Geometry: final body of the model. Coordinates: model frame, mm. Face numbers are marked on the shaded views. A direction names the side the tool comes from. Coordinates: 2 decimals unless noted, no trailing zeros. Order: outer loops, then holes, each group sorted by start corner. A loop starts at its lowest first (then second) coordinate and runs counter-clockwise, first axis right, second up. Notation, with made-up numbers: (-18, 79.25) - (11, 79.25) arc R34 ccw to (11, 116.25) - close; hole circle Ø8 at (-23.75, 87). An arc over 180 degrees is marked (long way). Use a Markdown table: item, result. Add a question column.
```python
from build123d import *

# Parameters (mm, degrees)
SKETCH1_W                                  = 128
SKETCH1_H                                  = 105
BOSS_EXTRUDE1_DEPTH                        = 3
SKETCH2_W                                  = 13.5
SKETCH2_H                                  = 105
BOSS_EXTRUDE2_DEPTH                        = 2.9
BOSS_EXTRUDE9_DEPTH                        = 7
FILLET2_R                                  = 1
CUT_EXTRUDE1_DEPTH                         = 7
SKETCH3_W                                  = 3
SKETCH3_H                                  = 95
BOSS_EXTRUDE10_DEPTH                       = 20
SKETCH11_R                                 = 1
CUT_EXTRUDE2_DEPTH                         = 20
SKETCH13_R                                 = 1
CUT_EXTRUDE3_DEPTH                         = 20
MIRROR1_AT_THE_SECOND_PLANE_COPY_1_SKETC_R = 1
MIRROR1_AT_THE_SECOND_PLANE_COPY_1_DEPTH   = 20
CUT_EXTRUDE8_DEPTH                         = 5
FILLET3_R                                  = 10


with BuildPart() as part:
    # Sketch1 → Boss-Extrude1 (new body)
    with BuildSketch(Plane(origin=(0, 0, 0), x_dir=(1, 0, 0), z_dir=(0, 1, 0))):
        Rectangle(SKETCH1_W, SKETCH1_H)
    extrude(amount=BOSS_EXTRUDE1_DEPTH)

    # Sketch2 → Boss-Extrude2 (add)
    with BuildSketch(Plane(origin=(0, 0, 0), x_dir=(1, 0, 0), z_dir=(0, 1, 0))):
        with Locations((-70.75, 0)):
            Rectangle(SKETCH2_W, SKETCH2_H)
        with Locations((70.75, 0)):
            Rectangle(SKETCH2_W, SKETCH2_H)
    extrude(amount=BOSS_EXTRUDE2_DEPTH)

    # Sketch5 → Boss-Extrude9 (add)
    with BuildSketch(Plane(origin=(0, 3, 0), x_dir=(1, 0, 0), z_dir=(0, 1, 0))):
        Polygon((-6, -18.5), (-6, -17.5), (-13, -17.5), (-13, 17.5), (13, 17.5), (13, -17.5), (6, -17.5), (6, -18.5), (14, -18.5), (14, 18.5), (-14, 18.5), (-14, -18.5), align=None)
    extrude(amount=BOSS_EXTRUDE9_DEPTH)

    # Fillet2
    fillet2_edges = [part.edges().sort_by_distance(p)[0] for p in [
        (13, 6.5, 17.5),
        (14, 6.5, 18.5),
        (14, 6.5, -18.5),
        (-14, 6.5, -18.5),
        (-14, 6.5, 18.5),
        (-13, 6.5, 17.5),
        (-13, 6.5, -17.5),
        (13, 6.5, -17.5),
    ]]
    fillet(fillet2_edges, radius=FILLET2_R)

    # Sketch10 → Cut-Extrude1 (cut)
    with BuildSketch(Plane(origin=(0, 3, 0), x_dir=(1, 0, 0), z_dir=(0, 1, 0))):
        with BuildLine():
            Line((-14, -17.381354556), (-45.915455387, -42.5))
            Line((-45.915455387, -42.5), (-6, -42.5))
            Line((-6, -42.5), (-6, -18.5))
            Line((-6, -18.5), (-13, -18.5))
            ThreePointArc((-13, -18.5), (-13.707106781, -18.207106781), (-14, -17.5))
            Line((-14, -17.5), (-14, -17.381354556))
        make_face()
        Polygon((-54, -6), (-54, -36.137163962), (-15.708074024, -6), align=None)
        with BuildLine():
            Line((6, -18.5), (6, -42.5))
            Line((6, -42.5), (45.915455387, -42.5))
            Line((45.915455387, -42.5), (14, -17.381354556))
            Line((14, -17.381354556), (14, -17.5))
            ThreePointArc((14, -17.5), (13.707106781, -18.207106781), (13, -18.5))
            Line((13, -18.5), (6, -18.5))
        make_face()
        Polygon((-54, 36.137163962), (-54, 6), (-15.708074024, 6), align=None)
        Polygon((15.708074024, -6), (54, -36.137163962), (54, -6), align=None)
        with BuildLine():
            Line((-6, 42.5), (-45.915455387, 42.5))
            Line((-45.915455387, 42.5), (-14, 17.381354556))
            Line((-14, 17.381354556), (-14, 17.5))
            ThreePointArc((-14, 17.5), (-13.707106781, 18.207106781), (-13, 18.5))
            Line((-13, 18.5), (-6, 18.5))
            Line((-6, 18.5), (-6, 42.5))
        make_face()
        Polygon((15.708074024, 6), (54, 6), (54, 36.137163962), align=None)
        with BuildLine():
            Line((45.915455387, 42.5), (6, 42.5))
            Line((6, 42.5), (6, 18.5))
            Line((6, 18.5), (13, 18.5))
            ThreePointArc((13, 18.5), (13.707106781, 18.207106781), (14, 17.5))
            Line((14, 17.5), (14, 17.381354556))
            Line((14, 17.381354556), (45.915455387, 42.5))
        make_face()
    extrude(amount=-CUT_EXTRUDE1_DEPTH, mode=Mode.SUBTRACT)

    # Sketch3 → Boss-Extrude10 (add)
    with BuildSketch(Plane(origin=(0, 0, 0), x_dir=(1, 0, 0), z_dir=(0, 1, 0))):
        with Locations((-79, 0)):
            Rectangle(SKETCH3_W, SKETCH3_H)
        with Locations((79, 0)):
            Rectangle(SKETCH3_W, SKETCH3_H)
    extrude(amount=BOSS_EXTRUDE10_DEPTH)

    # Sketch11 → Cut-Extrude2 (cut)
    with BuildSketch(Plane(origin=(0, 3, 0), x_dir=(1, 0, 0), z_dir=(0, 1, 0))):
        with Locations(Location((-63.3, -41, 0), (0, 0, 270))):
            Circle(SKETCH11_R)
        with Locations(Location((-63.3, -34.5, 0), (0, 0, 270))):
            Circle(SKETCH11_R)
        with Locations(Location((-63.3, 34.5, 0), (0, 0, 270))):
            Circle(SKETCH11_R)
        with Locations(Location((-63.3, 41, 0), (0, 0, 270))):
            Circle(SKETCH11_R)
        with Locations(Location((63.3, 41, 0), (0, 0, 270))):
            Circle(SKETCH11_R)
        with Locations(Location((63.3, 34.5, 0), (0, 0, 270))):
            Circle(SKETCH11_R)
        with Locations(Location((63.3, -34.5, 0), (0, 0, 270))):
            Circle(SKETCH11_R)
        with Locations(Location((63.3, -41, 0), (0, 0, 270))):
            Circle(SKETCH11_R)
    extrude(amount=-CUT_EXTRUDE2_DEPTH, mode=Mode.SUBTRACT)

    # Sketch13 → Cut-Extrude3 (cut)
    with BuildSketch(Plane(origin=(-77.5, 0, 0), x_dir=(0, 0, -1), z_dir=(1, 0, 0))):
        with Locations((-41, 14.842473729)):
            Circle(SKETCH13_R)
        with Locations((-34.5, 14.842473729)):
            Circle(SKETCH13_R)
    cut_extrude3 = extrude(amount=-CUT_EXTRUDE3_DEPTH, mode=Mode.SUBTRACT)

    # Mirror1: Cut-Extrude3 across plane
    add(cut_extrude3.mirror(Plane.XY), mode=Mode.SUBTRACT)

    # Mirror1 at the second plane: Cut-Extrude3 across plane
    add(cut_extrude3.mirror(Plane(origin=(0, 0, 0), x_dir=(0, 0, 1), z_dir=(1, 0, 0))), mode=Mode.SUBTRACT)

    # Mirror1 at the second plane copy 1 sketc → Mirror1 at the second plane copy 1 (cut)
    with BuildSketch(Plane.ZY.offset(-77.5)):
        with Locations((-41, 14.842473729)):
            Circle(MIRROR1_AT_THE_SECOND_PLANE_COPY_1_SKETC_R)
        with Locations((-34.5, 14.842473729)):
            Circle(MIRROR1_AT_THE_SECOND_PLANE_COPY_1_SKETC_R)
    extrude(amount=-MIRROR1_AT_THE_SECOND_PLANE_COPY_1_DEPTH, mode=Mode.SUBTRACT)

    # Sketch22 → Cut-Extrude8 (cut)
    with BuildSketch(Plane(origin=(0, 10, 0), x_dir=(1, 0, 0), z_dir=(0, 1, 0))):
        with BuildLine():
            Line((14, -17.5), (14, 17.5))
            ThreePointArc((14, 17.5), (13.707106781, 18.207106781), (13, 18.5))
            Line((13, 18.5), (-13, 18.5))
            ThreePointArc((-13, 18.5), (-13.707106781, 18.207106781), (-14, 17.5))
            Line((-14, 17.5), (-14, -17.5))
            ThreePointArc((-14, -17.5), (-13.707106781, -18.207106781), (-13, -18.5))
            Line((-13, -18.5), (-6, -18.5))
            Line((-6, -18.5), (-6, -17.5))
            Line((-6, -17.5), (-12, -17.5))
            ThreePointArc((-12, -17.5), (-12.707106781, -17.207106781), (-13, -16.5))
            Line((-13, -16.5), (-13, 16.5))
            ThreePointArc((-13, 16.5), (-12.707106781, 17.207106781), (-12, 17.5))
            Line((-12, 17.5), (12, 17.5))
            ThreePointArc((12, 17.5), (12.707106781, 17.207106781), (13, 16.5))
            Line((13, 16.5), (13, -16.5))
            ThreePointArc((13, -16.5), (12.707106781, -17.207106781), (12, -17.5))
            Line((12, -17.5), (6, -17.5))
            Line((6, -17.5), (6, -18.5))
            Line((6, -18.5), (13, -18.5))
            ThreePointArc((13, -18.5), (13.707106781, -18.207106781), (14, -17.5))
        make_face()
    extrude(amount=-CUT_EXTRUDE8_DEPTH, mode=Mode.SUBTRACT)

    # Fillet3
    # the kernel refuses this fillet: 10 mm, written as the material it takes off along each edge
    with BuildSketch(Plane(origin=(6, 5, 2.5), x_dir=(0, -1, 0), z_dir=(0, 0, 1)), Plane(origin=(-6, 5, 33.5), x_dir=(0, -1, 0), z_dir=(0, 0, -1))) as fillet3_piece_1:
        with BuildLine():
            CenterArc((10, 6), FILLET3_R, 180, 36.869897646)
            Line((0, 6), (-0.2, 6))
            Line((-0.2, 6), (-0.2, 0))
            Line((-0.2, 0), (0, -0.2))
            ThreePointArc((0, -0.2), (1, -0.2), (1.84, -0.12))
            Line((1.84, -0.12), (2, 0))
        make_face()
    extrude(amount=31, mode=Mode.SUBTRACT)


solid = part.part
```
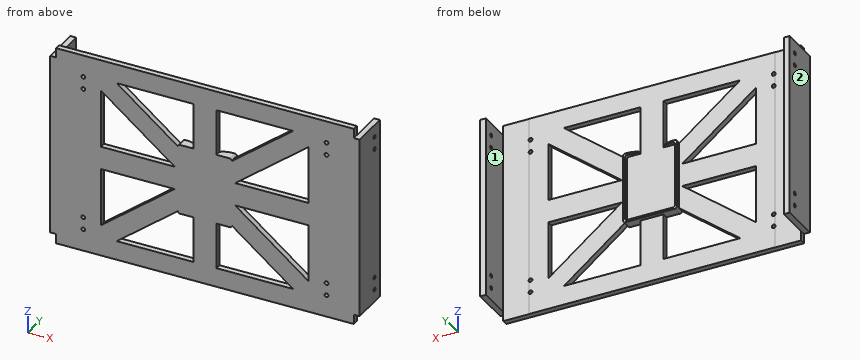
1) Pin query (flat end, axial travel): pin 1 (2.5 mm diameter, centred on x = -79.5, y = 9.5, fed in from +Z); pin 2 (1 mm diameter, centred on x = 55, z = 35.5, fed in from -Y); pin 3 (3 mm diameter, centred on y = 1, z = -50, fed in from -X); pin 4 (1.5 mm diameter, centred on x = 78.5, y = 8, fed in from -Z). Return the tip coordinate at first contact, or that it passes through.
2) Ray query, line 1 along Z through (x, y) = (-63.3, 1.65); line 2 along X through (y, z) = (11.25, -28.5); line 3 along Y through (x, z) = (78.45, 34.5). Return the intervals inside material, ascending.
3) Section A-A (y = 18). Return loops of the section in (x, z).
4) Section C-C (z = -3). Return loops of the section in (x, y), then the cut area to 3 significant figures.
5) Section D-D (z = -22). Return loops of the section in (x, y).
6) Set-up query: the marked faces 1 and 2. Return all of +Z, -Z, +X, -X, +Y, -Y with unobstructed straight access to the full face (end or side cutting, diameter ignored); none if empty.
7) Section B-B (x = 21). Return loops of the section in (y, z), then the cut area to 3 significant figures.
Values follow:
| question | item | result |
|---|---|---|
| 1 | pin 1 | stops at z = 47.5 |
| 1 | pin 2 | stops at y = 0 |
| 1 | pin 3 | stops at x = -77.5 |
| 1 | pin 4 | stops at z = -47.5 |
| 2 | line 1 | z = -52.5 to -42, -40 to -35.5, -33.5 to 33.5, 35.5 to 40, 42 to 52.5 |
| 2 | line 2 | x = -80.5 to -77.5, 77.5 to 80.5 |
| 2 | line 3 | y = 0 to 13.84, 15.84 to 20 |
| 3 | outline | (-80.5, -47.5) - (-77.5, -47.5) - (-77.5, 47.5) - (-80.5, 47.5) - close; (77.5, -47.5) - (80.5, -47.5) - (80.5, 47.5) - (77.5, 47.5) - close |
| 4 | outline | (-80.5, 0) - (80.5, 0) - (80.5, 20) - (77.5, 20) - (77.5, 2.9) - (64, 2.9) - (64, 3) - (14, 3) - (14, 5) - (13, 5) - (13, 3) - (-13, 3) - (-13, 5) - (-14, 5) - (-14, 3) - (-64, 3) - (-64, 2.9) - (-77.5, 2.9) - (-77.5, 20) - (-80.5, 20) - close |
| 4 | area | 586 mm² |
| 5 | outline | (-80.5, 0) - (-54, 0) - (-54, 3) - (-64, 3) - (-64, 2.9) - (-77.5, 2.9) - (-77.5, 20) - (-80.5, 20) - close; (-36.04, 0) - (-19.87, 0) - (-19.87, 3) - (-36.04, 3) - close; (-6, 0) - (6, 0) - (6, 3) - (-6, 3) - close; (19.87, 0) - (36.04, 0) - (36.04, 3) - (19.87, 3) - close; (54, 0) - (80.5, 0) - (80.5, 20) - (77.5, 20) - (77.5, 2.9) - (64, 2.9) - (64, 3) - (54, 3) - close |
| 6 | face 1 | +Z, -Z, +Y |
| 6 | face 2 | +Z, -Z, -X, +Y, -Y |
| 7 | outline | (0, -52.5) - (3, -52.5) - (3, -42.5) - (0, -42.5) - close; (0, -22.89) - (3, -22.89) - (3, -10.16) - (0, -10.16) - close; (0, -6) - (3, -6) - (3, 6) - (0, 6) - close; (0, 10.16) - (3, 10.16) - (3, 22.89) - (0, 22.89) - close; (0, 42.5) - (3, 42.5) - (3, 52.5) - (0, 52.5) - close |
| 7 | area | 172 mm² |
